Design review of the part built by this model. Coordinates are the model's own, in mm. A direction names the side the tool comes from. Round coordinates to 2 decimals unless told otherwise and drop trailing zeros. Write each loop counter-clockwise with the first axis right and the second up, starting at its lowest first coordinate (ties: lowest second). Pieces come first, ordered by that corner, then holes. Notation, with made-up numbers: M 6.5,47 L 19.5,47 A34 cw 19.5,82 Z; hole C 5,-39 d6. An arc over 180 degrees is marked long. One line per question, with ' | ' between items. Start each with the question number.
Item 1: Draft analysis for pull direction X (two halves, no side actions). For faces 1 (the face through (3, 3.175, 38)), 2 (the face through (3, 0, 37)), 3 (the face through (-204.788, 50, 106)), state which applies: released by +X, released by -X, zero draft, split by the parting line, or undercut.
Item 2: Machinability: for faces 4 (the face through (65.844, 51.699, 173.474)), 5 (the face through (-203.2, 52, 103)), 6 (the face through (-49.212, 50, 178)), which of the approach directions +Z, -Z, +X, -X, +Y, -Y give a long, thin tool a straight path to every point of the face, cutting with its end or side? Answer none if there is none.
Item 3: Add section A-A, the plane x = 0. State the section outline as (y, z) points (1 decimal), and give its area (3 significant figures).
Item 4: Add section B-B, the plane z = 59.5. State the section outline as (x, y) points (1 decimal).
Item 5: For L1, parallel to X at y = 1, z = 0; L2, parallel to X at y = 30, z = 190.5; L3, parallel to Y at x = 87.5, z = 119 (3 decimals), list the stretches that pass through material, from the lowest coordinate up.
Item 6: Add section D-D, the plane x = 165. State the section outline as (y, z) points (3 decimals), and give its area (3 significant figures).
Item 7: Insertion check: pin 1 Ø5 at (x, z) = (46.5, 84) entering from -Y; pin 2 Ø3.5 at (y, z) = (1.5, 248.5) entering from +X; pin 3 Ø3 at (x, y) = (-64, 80) entering from -Z; pin 4 Ø1.7 at (x, y) = (-50, 36.5) entering from +Z. Each pin has a flat end and moves straight along its axis. Give the tip position at first contact, or say it passes through.
```python
from build123d import *

# Parameters (mm, degrees)
BOSS_EXTRUDE1_DEPTH = 101.6
BOSS_EXTRUDE2_DEPTH = 3.175
SKETCH3_R           = 14.2875
CUT_EXTRUDE1_DEPTH  = 4.175


with BuildPart() as part:
    # Sketch1 → Boss-Extrude1 (new body)
    with BuildSketch(Plane(origin=(0, 0, 0), x_dir=(1, 0, 0), z_dir=(0, 1, 0))):
        with BuildLine():
            Line((-203.2, 0), (-203.2, -209.748302875))
            Line((-203.2, -209.748302875), (-204.7875, -209.748302875))
            Line((-204.7875, -209.748302875), (-204.7875, 0))
            ThreePointArc((-204.7875, 0), (57.689818519, 196.493778516), (172.284391551, -110.706858794))
            ThreePointArc((172.284391551, -110.706858794), (73.781728286, -174.14050958), (-38.721251967, -141.434513854))
            ThreePointArc((-38.721251967, -141.434513854), (-45.510666818, -140.476846169), (-49.2125, -146.248302875))
            Line((-49.2125, -146.248302875), (-49.2125, -209.748302875))
            Line((-49.2125, -209.748302875), (-50.8, -209.748302875))
            Line((-50.8, -209.748302875), (-50.8, -196.747553987))
            Line((-50.8, -196.747553987), (-50.8, -133.791705405))
            ThreePointArc((-50.8, -133.791705405), (-49.219066452, -131.439729313), (-46.444258629, -132.015562597))
            ThreePointArc((-46.444258629, -132.015562597), (67.592808645, -173.307075278), (170.948853632, -109.848666091))
            ThreePointArc((170.948853632, -109.848666091), (57.242610623, 194.970570931), (-203.2, 0))
        make_face()
    extrude(amount=BOSS_EXTRUDE1_DEPTH)

    # Sketch2 → Boss-Extrude2 (add)
    with BuildSketch(Plane(origin=(0, 0, 0), x_dir=(1, 0, 0), z_dir=(0, 1, 0))):
        with BuildLine():
            Line((-50.8, -133.791705405), (-50.8, -286.191705405))
            Line((-50.8, -286.191705405), (-203.2, -286.191705405))
            Line((-203.2, -286.191705405), (-203.2, 0))
            ThreePointArc((-203.2, 0), (57.242610623, 194.970570931), (170.948853632, -109.848666091))
            ThreePointArc((170.948853632, -109.848666091), (67.592808645, -173.307075278), (-46.444258629, -132.015562597))
            ThreePointArc((-46.444258629, -132.015562597), (-49.219066452, -131.439729313), (-50.8, -133.791705405))
        make_face()
    extrude(amount=BOSS_EXTRUDE2_DEPTH)

    # Sketch3 → Cut-Extrude1 (cut, through all)
    with BuildSketch(Plane(origin=(0, 3.175, 0), x_dir=(1, 0, 0), z_dir=(0, 1, 0))):
        Circle(SKETCH3_R)
    extrude(amount=-CUT_EXTRUDE1_DEPTH, mode=Mode.SUBTRACT)


solid = part.part
```
Computed values:
1) face 1: undercut | face 2: zero draft | face 3: released by -X
2) face 4: +Y | face 5: +Z, +Y | face 6: +Z, +Y, -Y
3) outline: M 0,-204.8 L 101.6,-204.8 L 101.6,-203.2 L 3.2,-203.2 L 3.2,-14.3 L 0,-14.3 Z; M 0,14.3 L 3.2,14.3 L 3.2,163.4 L 101.6,163.4 L 101.6,165.1 L 0,165.1 Z | area: 1,410 mm^2
4) outline: M -204.8,0 L 196,0 L 196,101.6 L 194.3,101.6 L 194.3,3.2 L -203.2,3.2 L -203.2,101.6 L -204.8,101.6 Z
5) L1: x = -204.79 to -14.29, 14.29 to 204.79 | L2: x = -204.79 to -203.2, -50.8 to -49.21 | L3: y = 0 to 3.175
6) outline: M 0,-121.297 L 101.6,-121.297 L 101.6,-118.597 L 3.175,-118.597 L 3.175,118.389 L 101.6,118.389 L 101.6,121.002 L 0,121.002 Z | area: 1,290 mm^2
7) pin 1: stops at y = 0 | pin 2: stops at x = -50.8 | pin 3: stops at z = -195.02 | pin 4: stops at z = 209.75
